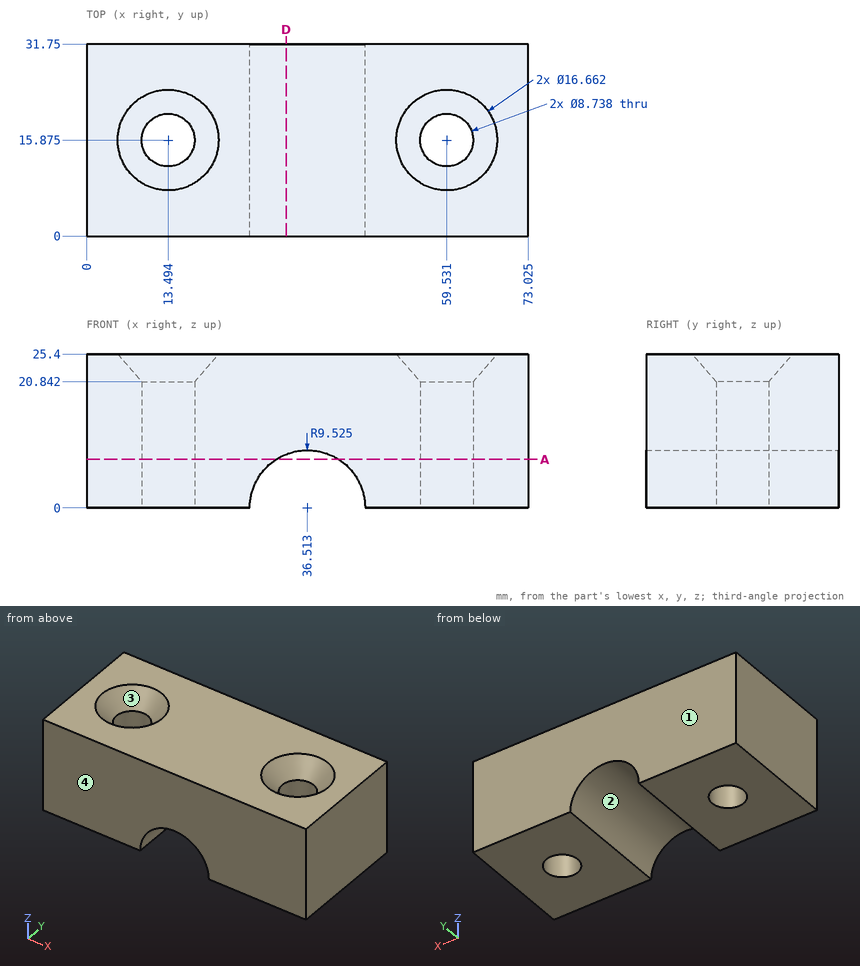
Part print with two shaded views. Sizes in mm from the minimum x, y, z corner. Round coordinates to 2 decimals unless told otherwise and drop trailing zeros. Loops run counter-clockwise (first coordinate to the right, second up) from the corner with the lowest first, then second, coordinate; pieces in that order, holes last. Notation, with made-up numbers: (-31, 73.25) - (-7, 73.25) arc R20 cw to (-7, 110.25) - close; hole circle Ø4 at (72, -4.5). An arc over 180 degrees is marked (long way). Put each result on its own line as item: value.
1. Slice it at A-A on z = 8. Give the number of separate pieces and of enclosed holes in the cut face, and give its area (3 significant figures).
Geometry check:
separate pieces: 2
enclosed holes: 2
area: 1,870 mm²
2. Two-plate mould, pull along Y, no slides. Class the marked faces 1, 2, 3 and 4: released by +Y, released by -Y, zero draft, split by the parting line, or undercut.
Geometry check:
face 1: released by +Y
face 2: zero draft
face 3: undercut
face 4: released by -Y
3. Slice it at D-D on x = 33. List the corners of the cut face in (y, z).
Geometry check:
outline: (0, 8.85) - (31.75, 8.85) - (31.75, 25.4) - (0, 25.4) - close
4. Wall check: line 1 (X direction, y = 16.5, z = 4.25) (1 decimal); line 2 (X direction, y = 13.5, z = 21) (1 decimal); line 3 (Y direction, x = 60, z = 9.75). Give the ranges that are in metal, low to high.
Geometry check:
line 1: 0 to 9.2, 17.8 to 28, 45 to 55.2, 63.9 to 73
line 2: 0 to 9.7, 17.3 to 55.7, 63.4 to 73
line 3: 0 to 11.53, 20.22 to 31.75
5. Pin check, flat tip, straight feed: P1, Ø14, axis at x = 59.53, y = 15.88, coming from the +Z side (1 decimal). Stop position of the tip, or through.
Geometry check:
P1: z = 23.9
